```python
from build123d import *

# Parameters (mm, degrees)
SKETCH1_R           = 25
BOSS_EXTRUDE1_DEPTH = 20
FILLET3_R           = 1
SKETCH2_R           = 3
CUT_EXTRUDE1_DEPTH  = 12.5


with BuildPart() as part:
    # Sketch1 → Boss-Extrude1 (new body)
    with BuildSketch(Plane(origin=(0, 0, 0), x_dir=(1, 0, 0), z_dir=(0, 1, 0))):
        with Locations(Location((0, 0, 0), (0, 0, 270))):
            Circle(SKETCH1_R)
    extrude(amount=-BOSS_EXTRUDE1_DEPTH)

    # Fillet3
    fillet3_edges = [part.edges().sort_by_distance(p)[0] for p in [
        (0, 0, -25),
        (0, -20, -25),
    ]]
    fillet(fillet3_edges, radius=FILLET3_R)

    # Sketch2 → Cut-Extrude1 (cut)
    with BuildSketch(Plane.XZ.offset(20)):
        with Locations(Location((0, 0, 0), (0, 0, 270))):
            Circle(SKETCH2_R)
    extrude(amount=-CUT_EXTRUDE1_DEPTH, mode=Mode.SUBTRACT)


solid = part.part
```
The model under review builds one solid part; all positions refer to its coordinate system, in mm. Coordinates: 2 decimals unless noted, no trailing zeros. Write each loop counter-clockwise with the first axis right and the second up, starting at its lowest first coordinate (ties: lowest second). Pieces come first, ordered by that corner, then holes.
1) The part is to be moulded in two halves that separate along Z. For faces 1 (the face through (0, -20, 5)), 2 (the face through (7.509, -9.874, 23.846)), 3 (the face through (0.9, -13.84, -2.86)), 4 (the face through (0, -7.5, 0)), say which applies: pulls with the +Z half, pulls with the -Z half, needs draft (parallel to the pull), parting line crosses it, or undercut.
2) To check wall thickness, follow probe 1 along X at (y, z) = (-11.75, 0); probe 2 along Z at (x, y) = (7, -15.5); probe 3 along X at (y, z) = (-15.75, 5.5). State the ranges of each line that lie inside material, in increasing order.
3) We need section D-D on y = -4. State the section outline as (x, z) points.
4) We need section A-A on x = 0. State the section outline as (y, z) points, then the cut area to 3 significant figures.
5) We need section C-C on y = -11.5. State the section outline as (x, z) points, then the cut area to 3 significant figures.
6) We need section B-B on z = 0. State the section outline as (x, y) points, then the cut area to 3 significant figures.
7) Clearance check with flat-ended pins moving along their axes: pin 1 Ø3 at (x, y) = (5.5, -18) entering from -Z; pin 2 Ø1.8 at (x, z) = (0.5, 0) entering from -Y; pin 3 Ø8 at (x, y) = (-20, -13) entering from -Z. State where each tip first meets the part, or that it passes through.
Answer list:
1. face 1: needs draft
1. face 2: parting line crosses it
1. face 3: undercut
1. face 4: undercut
2. probe 1: x = -25 to -3, 3 to 25
2. probe 2: z = -24 to 24
2. probe 3: x = -24.39 to 24.39
3. outline: circle Ø50 at (0, 0)
4. outline: (-20, -24) arc R1 ccw to (-19, -25) - (-1, -25) arc R1 ccw to (0, -24) - (0, 24) arc R1 ccw to (-1, 25) - (-19, 25) arc R1 ccw to (-20, 24) - (-20, 3) - (-7.5, 3) - (-7.5, -3) - (-20, -3) - close
4. area: 924 mm2
5. outline: circle Ø50 at (0, 0); hole circle Ø6 at (0, 0)
5. area: 1,940 mm2
6. outline: (-25, -19) arc R1 ccw to (-24, -20) - (-3, -20) - (-3, -7.5) - (3, -7.5) - (3, -20) - (24, -20) arc R1 ccw to (25, -19) - (25, -1) arc R1 ccw to (24, 0) - (-24, 0) arc R1 ccw to (-25, -1) - close
6. area: 924 mm2
7. pin 1: stops at z = -24.68
7. pin 2: stops at y = -7.5
7. pin 3: stops at z = -19.21
